Build history of the part. All positions in model axes, mm. A direction names the side the tool comes from. Give positions to 0.01 mm unless a question says otherwise; leave off trailing zeros. Loops run counter-clockwise (first coordinate to the right, second up) from the corner with the lowest first, then second, coordinate; pieces in that order, holes last. Notation, with made-up numbers: M -21,73 L -17,73 A32 ccw -17,109 Z; hole C 79,33 d10. An arc over 180 degrees is marked long. Answer as a JSON object with one key per item and string values. Group by question number.
1. 3-axis set-ups, long thin cutter, end or side, ignore diameter. For faces 1 (the face through (2, -4, 12)), 2 (the face through (1, -5, 5)), 3 (the face through (0.99, -12.76, -0.16)): which of +Z, -Z, +X, -X, +Y, -Y reach the whole face in a straight line?
2. Mould opens along Y. For faces 4 (the face through (0, 4, 12)), 5 (the face through (4.03, -11.99, 0.53)), 6 (the face through (1.49, -5.5, 2.86)) say: released by +Y, released by -Y, zero draft, split by the parting line, or undercut.
3. Drill centre lines: line 1 along Y through (x, z) = (1.9, -7.5); line 2 along Y through (x, z) = (0.85, -14); line 3 along Z through (x, y) = (4.35, -1). Where is each one in solid material? Low to high. Write a range as [from, to].
4. Slice it at C-C (y = 0). List the corners of the cut face in (x, z), then the cut area to 3 significant figures.
5. Slice it at D-D (x = 4.6). List the corners of the cut face in (y, z), then the cut area to 3 significant figures.
6. Slice it at A-A (y = -14). List the corners of the cut face in (x, z).
7. Drop flat-ended pins along their axis: pin 1 Ø5.5 at (y, z) = (4.5, 1) entering from +X; pin 2 Ø20 at (y, z) = (0, 0) entering from -X; pin 3 Ø2 at (y, z) = (-14, 0) entering from -X; pin 4 Ø2 at (x, y) = (3.5, -9) entering from +Z. Give the stop position or say it passes through.
from build123d import *

# Parameters (mm, degrees)
CUT_EXTRUDE3_REACH = 8
SKETCH4_R          = 1.25
SKETCH2_R          = 12
CUT_EXTRUDE4_DEPTH = 1
CUT_EXTRUDE5_REACH = 7
SKETCH5_R          = 6.2


with BuildPart() as part:
    # Sketch1 → Revolve1 (revolve)
    with BuildSketch(Plane.XY):
        Polygon((0, 0), (0, 17), (2, 17), (2, 12), (6, 12), (6, 10), (2, 9), (2, 0), align=None)
    revolve(axis=Axis((0, 0, 0), (1, 0, 0)))

    # Sketch4 → Cut-Extrude3 (cut, up to next)
    with BuildSketch(Plane.ZY, mode=Mode.PRIVATE) as cut_extrude3_sk1:
        with Locations((0, 14)):
            Circle(SKETCH4_R)
    cut_extrude3_tool1 = extrude(cut_extrude3_sk1.sketch, amount=-CUT_EXTRUDE3_REACH, mode=Mode.PRIVATE) & part.part
    add(cut_extrude3_tool1.solids().sort_by_distance((0, 14, 0))[0], mode=Mode.SUBTRACT)
    # Sketch4 → Cut-Extrude3 (cut, up to next)
    with BuildSketch(Plane.ZY, mode=Mode.PRIVATE) as cut_extrude3_sk2:
        with Locations((14, 0)):
            Circle(SKETCH4_R)
    cut_extrude3_tool2 = extrude(cut_extrude3_sk2.sketch, amount=-CUT_EXTRUDE3_REACH, mode=Mode.PRIVATE) & part.part
    add(cut_extrude3_tool2.solids().sort_by_distance((0, 0, 14))[0], mode=Mode.SUBTRACT)
    # Sketch4 → Cut-Extrude3 (cut, up to next)
    with BuildSketch(Plane.ZY, mode=Mode.PRIVATE) as cut_extrude3_sk3:
        with Locations((0, -14)):
            Circle(SKETCH4_R)
    cut_extrude3_tool3 = extrude(cut_extrude3_sk3.sketch, amount=-CUT_EXTRUDE3_REACH, mode=Mode.PRIVATE) & part.part
    add(cut_extrude3_tool3.solids().sort_by_distance((0, -14, 0))[0], mode=Mode.SUBTRACT)
    # Sketch4 → Cut-Extrude3 (cut, up to next)
    with BuildSketch(Plane.ZY, mode=Mode.PRIVATE) as cut_extrude3_sk4:
        with Locations((-14, 0)):
            Circle(SKETCH4_R)
    cut_extrude3_tool4 = extrude(cut_extrude3_sk4.sketch, amount=-CUT_EXTRUDE3_REACH, mode=Mode.PRIVATE) & part.part
    add(cut_extrude3_tool4.solids().sort_by_distance((0, 0, -14))[0], mode=Mode.SUBTRACT)

    # Sketch2 → Cut-Extrude4 (cut)
    with BuildSketch(Plane.ZY):
        Circle(SKETCH2_R)
    extrude(amount=-CUT_EXTRUDE4_DEPTH, mode=Mode.SUBTRACT)

    # Sketch5 → Cut-Extrude5 (cut, up to next)
    with BuildSketch(Plane.ZY.offset(-1), mode=Mode.PRIVATE) as cut_extrude5_sk1:
        Circle(SKETCH5_R)
    cut_extrude5_tool1 = extrude(cut_extrude5_sk1.sketch, amount=-CUT_EXTRUDE5_REACH, mode=Mode.PRIVATE) & part.part
    add(cut_extrude5_tool1.solids().sort_by_distance((1, 0, 0))[0], mode=Mode.SUBTRACT)


solid = part.part
Established:
{
 "1": {"face 1": "+X", "face 2": "-X", "face 3": "+X, -X"},
 "2": {"face 4": "zero draft", "face 5": "split by the parting line", "face 6": "undercut"},
 "3": {"line 1": "y = [-15.26, 15.26]", "line 2": "y = [-9.64, -1.25], [1.25, 9.64]", "line 3": "z = [-11.96, -9.54], [9.54, 11.96]"},
 "4": {"outline": "M 0,-17 L 2,-17 L 2,-15.25 L 0,-15.25 Z; M 0,-12.75 L 2,-12.75 L 2,-12 L 6,-12 L 6,-10 L 2,-9 L 2,-6.2 L 1,-6.2 L 1,-12 L 0,-12 Z; M 0,12 L 1,12 L 1,6.2 L 2,6.2 L 2,9 L 6,10 L 6,12 L 2,12 L 2,12.75 L 0,12.75 Z; M 0,15.25 L 2,15.25 L 2,17 L 0,17 Z", "area": "41.6 mm^2"},
 "5": {"outline": "C 0,0 d24; hole C 0,0 d19.3", "area": "160 mm^2"},
 "6": {"outline": "M 0,-9.64 L 2,-9.64 L 2,-1.25 L 0,-1.25 Z; M 0,1.25 L 2,1.25 L 2,9.64 L 0,9.64 Z"},
 "7": {"pin 1": "stops at x = 2", "pin 2": "stops at x = 1", "pin 3": "passes through", "pin 4": "stops at z = 8.94"}
}
